Could you check a few things on this model? Use its own coordinates, in mm. Face numbers are marked on the shaded views. Give positions to 0.01 mm unless a question says otherwise; leave off trailing zeros. Loops run counter-clockwise (first coordinate to the right, second up) from the corner with the lowest first, then second, coordinate; pieces in that order, holes last.
1. Thinking about a two-plate mould opening in X: for the marked faces 1, 2 and 3, which applies, +X half, -X half, draft (parallel to the pull), parting line (faces both ways), or undercut?
2. Imagine slicing it at C-C (y = 1). List the corners of the cut face in (x, z) for me (3 decimals).
3. Imagine slicing it at B-B (x = -1.5). List the corners of the cut face in (y, z) for me (3 decimals).
4. Imagine slicing it at D-D (z = 8). List the corners of the cut face in (x, y) for me (3 decimals), plus the area to 3 significant figures.
5. For P1, Ø1.5, axis at y = -2, z = 15, coming from the -X side; P2, Ø2, axis at x = 1, y = 1, coming from the +Z side; P3, Ø3, axis at x = -1, y = 1.5, coming from the +Z side, each with a flat end and sliding along its axis, tell me the tip position at first contact or that it passes through.
6. Imagine slicing it at A-A (z = 13.25). List the corners of the cut face in (x, y) for me (3 decimals), plus the area to 3 significant figures.
7. I need wall thicknesses on line 1 along Y through (x, z) = (0, 15) (3 decimals); line 2 along Y through (x, z) = (1.5, 1) (3 decimals); line 3 along X through (y, z) = (1.75, 15.25). Which ranges of each line are inside material? Lowest first, please.
```python
from build123d import *

# Parameters (mm, degrees)
SKETCH1_R           = 3.875
SKETCH1_R_2         = 2.615
BOSS_EXTRUDE1_DEPTH = 22
BOSS_EXTRUDE2_DEPTH = 10
SKETCH4_W           = 7.75
SKETCH4_H           = 7.75
BOSS_EXTRUDE3_DEPTH = 5


with BuildPart() as part:
    # Sketch1 → Boss-Extrude1 (new body)
    with BuildSketch(Plane.XY):
        Circle(SKETCH1_R)
        Circle(SKETCH1_R_2, mode=Mode.SUBTRACT)
    extrude(amount=BOSS_EXTRUDE1_DEPTH)

    # Sketch2 → Boss-Extrude2 (add)
    with BuildSketch(Plane.XY.offset(10)):
        with BuildLine():
            Line((0, 3.875), (-3.875, 3.875))
            Line((-3.875, 3.875), (-3.875, 0))
            ThreePointArc((-3.875, 0), (-2.740038777, 2.740038777), (0, 3.875))
        make_face()
        with BuildLine():
            ThreePointArc((0, -3.875), (-2.740038777, -2.740038777), (-3.875, 0))
            Line((-3.875, 0), (-3.875, -3.875))
            Line((-3.875, -3.875), (0, -3.875))
        make_face()
        with BuildLine():
            Line((3.875, 3.875), (0, 3.875))
            ThreePointArc((0, 3.875), (2.740038777, 2.740038777), (3.875, 0))
            Line((3.875, 0), (3.875, 3.875))
        make_face()
        with BuildLine():
            Line((3.875, -3.875), (3.875, 0))
            ThreePointArc((3.875, 0), (2.740038777, -2.740038777), (0, -3.875))
            Line((0, -3.875), (3.875, -3.875))
        make_face()
    extrude(amount=-BOSS_EXTRUDE2_DEPTH)

    # Sketch4 → Boss-Extrude3 (add)
    with BuildSketch(Plane(origin=(0, 0, 0), x_dir=(-1, 0, 0), z_dir=(0, 0, -1))):
        Rectangle(SKETCH4_W, SKETCH4_H)
    extrude(amount=BOSS_EXTRUDE3_DEPTH)


solid = part.part
```
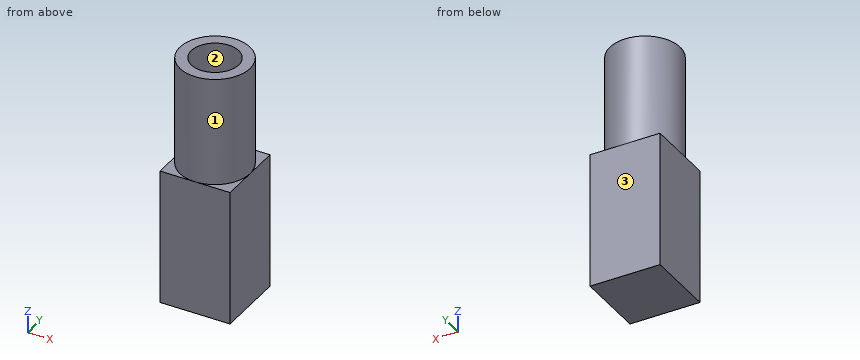
Derived:
1. face 1: parting line
1. face 2: undercut
1. face 3: draft
2. outline: (-3.875, -5) - (3.875, -5) - (3.875, 10) - (3.744, 10) - (3.744, 22) - (2.416, 22) - (2.416, 0) - (-2.416, 0) - (-2.416, 22) - (-3.744, 22) - (-3.744, 10) - (-3.875, 10) - close
3. outline: (-3.875, -5) - (3.875, -5) - (3.875, 10) - (3.573, 10) - (3.573, 22) - (2.142, 22) - (2.142, 0) - (-2.142, 0) - (-2.142, 22) - (-3.573, 22) - (-3.573, 10) - (-3.875, 10) - close
4. outline: (-3.875, -3.875) - (3.875, -3.875) - (3.875, 3.875) - (-3.875, 3.875) - close; hole circle Ø5.23 at (0, 0)
4. area: 38.6 mm2
5. P1: stops at x = -3.67
5. P2: stops at z = 0
5. P3: stops at z = 22
6. outline: circle Ø7.75 at (0, 0); hole circle Ø5.23 at (0, 0)
6. area: 25.7 mm2
7. line 1: y = -3.875 to -2.615, 2.615 to 3.875
7. line 2: y = -3.875 to -2.142, 2.142 to 3.875
7. line 3: x = -3.46 to -1.94, 1.94 to 3.46
